For this review, take the finished solid that the model builds, in its own axes (mm). Face numbers are marked on the shaded views. A direction names the side the tool comes from. Give positions to 0.01 mm unless a question says otherwise; leave off trailing zeros. Loops run counter-clockwise (first coordinate to the right, second up) from the corner with the lowest first, then second, coordinate; pieces in that order, holes last. Notation, with made-up numbers: (-27.5, 54.25) - (28.5, 54.25) arc R25 ccw to (28.5, 84.25) - close; hole circle Ø11 at (-39.5, 9.5). An arc over 180 degrees is marked (long way). Answer in a Markdown table with one row per item.
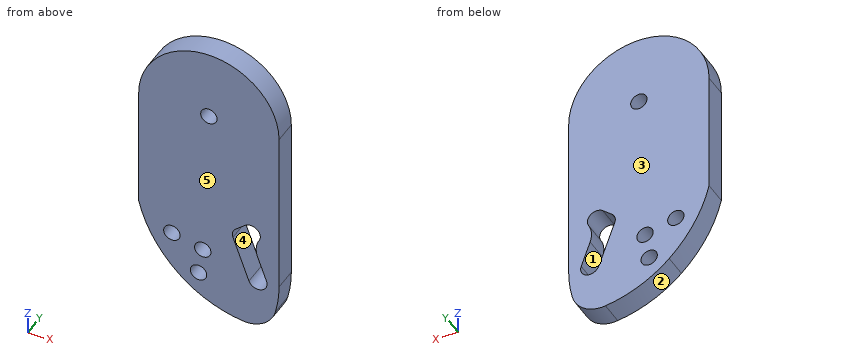
```python
from build123d import *

# Parameters (mm, degrees)
SKETCH1_R           = 1.75
BOSS_EXTRUDE1_DEPTH = 5
FILLET1_R           = 5
CUT_EXTRUDE1_DEPTH  = 10
SKETCH3_R           = 1.75
CUT_EXTRUDE2_DEPTH  = 10


with BuildPart() as part:
    # Sketch1 → Boss-Extrude1 (new body)
    with BuildSketch(Plane(origin=(0, 0, 0), x_dir=(1, 0, 0), z_dir=(0, 1, 0))):
        with BuildLine():
            Line((-15, 0), (-15, 50))
            ThreePointArc((-15, 50), (0, 65), (15, 50))
            Line((15, 50), (15, 0))
            ThreePointArc((15, 0), (0, -15), (-15, 0))
        make_face()
        Circle(SKETCH1_R, mode=Mode.SUBTRACT)
        with BuildLine():
            Line((12.324500118, 35.6706981), (9.383268849, 27.589731606))
            Line((9.383268849, 27.589731606), (10.285575219, 26.832606664))
            ThreePointArc((10.285575219, 26.832606664), (10.532088886, 24.014942558), (7.714424781, 23.768428891))
            Line((7.714424781, 23.768428891), (5.739338223, 25.425723293))
            ThreePointArc((5.739338223, 25.425723293), (5.09306179, 26.440174089), (5.145528201, 27.641852466))
            Line((5.145528201, 27.641852466), (8.565729634, 37.038778674))
            ThreePointArc((8.565729634, 37.038778674), (11.129155163, 38.234123628), (12.324500118, 35.6706981))
        make_face(mode=Mode.SUBTRACT)
    extrude(amount=BOSS_EXTRUDE1_DEPTH)

    # Fillet1
    fillet1_edges = [part.edges().sort_by_distance(p)[0] for p in [
        (9.383268849, 2.5, -27.589731606),
    ]]
    fillet(fillet1_edges, radius=FILLET1_R)

    # Sketch2 → Cut-Extrude1 (cut)
    with BuildSketch(Plane(origin=(0, 5, 0), x_dir=(1, 0, 0), z_dir=(0, 1, 0))):
        with BuildLine():
            Line((-15, 26.324644949), (-40.925594741, 69.238213195))
            Line((-40.925594741, 69.238213195), (-58.771967888, 111.080687023))
            Line((-58.771967888, 111.080687023), (39.28439299, 102.825794629))
            Line((39.28439299, 102.825794629), (15, 36.046990739))
            ThreePointArc((15, 36.046990739), (14.81014445, 39.245839168), (14.243243524, 42.399773179))
            ThreePointArc((14.243243524, 42.399773179), (11.621838426, 46.208407589), (7.127072402, 47.292169164))
            ThreePointArc((7.127072402, 47.292169164), (-0.175202385, 45.163669538), (-6.484026655, 40.9148504))
            ThreePointArc((-6.484026655, 40.9148504), (-11.826766868, 34.252893813), (-15, 26.324644949))
        make_face()
    extrude(amount=-CUT_EXTRUDE1_DEPTH, mode=Mode.SUBTRACT)

    # Sketch3 → Cut-Extrude2 (cut)
    with BuildSketch(Plane(origin=(0, 5, 0), x_dir=(1, 0, 0), z_dir=(0, 1, 0))):
        with Locations((-1.301778952, 33.126107378)):
            Circle(SKETCH3_R)
        with Locations((-2.207127715, 39.057409395)):
            Circle(SKETCH3_R)
        with Locations((-7.905919506, 31.519764857)):
            Circle(SKETCH3_R)
    extrude(amount=-CUT_EXTRUDE2_DEPTH, mode=Mode.SUBTRACT)


solid = part.part
```
1. We need section B-B, the plane y = 3.4. Count the separate pieces of the cut face and the enclosed holes in it, and give its area (3 significant figures).
Values:
| item | result |
|---|---|
| separate pieces | 1 |
| enclosed holes | 5 |
| area | 1,520 mm^2 |
2. Clearance check with flat-ended pins moving along their axes: pin 1 (1 mm diameter, centred on x = -4, y = 1, fed in from -Z); pin 2 (1 mm diameter, centred on x = 11, y = 3.5, fed in from +Z). State where each tip first meets the part, or that it passes through.
Values:
| item | result |
|---|---|
| pin 1 | stops at z = -43.28 |
| pin 2 | stops at z = 10.71 |
3. Wall thickness on line 1 (Z direction, x = -1, y = 0.75); line 2 (Z direction, x = 0, y = 4.6); line 3 (X direction, y = 4.3, z = -30): over which ranges is each line inside the solid? List them lowest first. Write a range as [from, to].
Values:
| item | result |
|---|---|
| line 1 | z = [-44.76, -40.32], [-37.79, -34.85], [-31.4, -1.44], [1.44, 14.97] |
| line 2 | z = [-45.24, -34.3], [-31.96, -1.75], [1.75, 15] |
| line 3 | x = [-13.87, -8.77], [-7.04, 6], [10.28, 15] |
4. Mouldability with a two-part tool opening along X and no side actions: class the marked faces 1, 2 and 3 as released by +X, released by -X, zero draft, split by the parting line, or undercut.
Values:
| item | result |
|---|---|
| face 1 | undercut |
| face 2 | released by -X |
| face 3 | zero draft |
5. For the marked faces 4 and 5, list the 3-axis set-ups (+Z, -Z, +X, -X, +Y, -Y) from which the entire face can be reached by the end or side of a thin tool; tool diameter is ignored.
Values:
| item | result |
|---|---|
| face 4 | +Y, -Y |
| face 5 | +Z, -Z, +X, -X, -Y |
6. We need section A-A, the plane x = 3. Give the boundary of the cut face in (y, z), and give its area (3 significant figures).
Values:
| item | result |
|---|---|
| outline | (0, -46.39) - (5, -46.39) - (5, 14.7) - (0, 14.7) - close |
| area | 305 mm^2 |
7. We need section C-C, the plane z = 9.5. Give the boundary of the cut face in (x, y), and give its area (3 significant figures).
Values:
| item | result |
|---|---|
| outline | (-11.61, 0) - (11.61, 0) - (11.61, 5) - (-11.61, 5) - close |
| area | 116 mm^2 |
